Could you check a few things on this model? Use its own coordinates, in mm. A direction names the side the tool comes from. Round coordinates to 2 decimals unless told otherwise and drop trailing zeros. Order: outer loops, then holes, each group sorted by start corner. A loop starts at its lowest first (then second) coordinate and runs counter-clockwise, first axis right, second up. Notation, with made-up numbers: (85, 69.5) - (119, 69.5) arc R20 ccw to (119, 80.5) - close; hole circle Ø7 at (-11.5, 79). An arc over 180 degrees is marked (long way). Return JSON: item names as keys, results as strings. Group by question number.
from build123d import *

# Parameters (mm, degrees)
SKETCH1_W           = 95.25
SKETCH1_H           = 79.375
SKETCH1_W_2         = 73.025
SKETCH1_H_2         = 28.575
BOSS_EXTRUDE1_DEPTH = 3.2
SKETCH2_W           = 95.25
SKETCH2_H           = 79.375
SKETCH2_W_2         = 88.85
SKETCH2_H_2         = 72.975
EXTRUDE_THIN1_DEPTH = 15.24
SKETCH3_R           = 4.064
CUT_EXTRUDE1_DEPTH  = 74.161631893


with BuildPart() as part:
    # Sketch1 → Boss-Extrude1 (new body)
    with BuildSketch(Plane(origin=(0, 0, 0), x_dir=(1, 0, 0), z_dir=(0, 1, 0))):
        with Locations((0, -12.7)):
            Rectangle(SKETCH1_W, SKETCH1_H)
        Rectangle(SKETCH1_W_2, SKETCH1_H_2, mode=Mode.SUBTRACT)
    extrude(amount=BOSS_EXTRUDE1_DEPTH)

    # Sketch2 → Extrude-Thin1 (add)
    with BuildSketch(Plane.XZ):
        with Locations((0, 12.7)):
            Rectangle(SKETCH2_W, SKETCH2_H)
        with Locations((0, 12.7)):
            Rectangle(SKETCH2_W_2, SKETCH2_H_2, mode=Mode.SUBTRACT)
    extrude(amount=EXTRUDE_THIN1_DEPTH)

    # Sketch3 → Cut-Extrude1 (cut, through all)
    with BuildSketch(Plane(origin=(0, 3.2, 0), x_dir=(1, 0, 0), z_dir=(0, 1, 0))):
        with Locations(Location((38.1, -30.1625, 0), (0, 0, 270))):
            Circle(SKETCH3_R)
        with Locations(Location((38.1, -42.8625, 0), (0, 0, 270))):
            Circle(SKETCH3_R)
    extrude(amount=-CUT_EXTRUDE1_DEPTH, mode=Mode.SUBTRACT)


solid = part.part
1) For faces 1 (the flat face through (-36.512, 2, 0)), 2 (the flat face through (-1, 0, 20)), 3 (the flat face through (47.625, -6, 12)), which set-ups out of +Z, -Z, +X, -X, +Y, -Y let a thin tool reach every point of the face, with its end or its side?
2) I want a section at A-A, the plane z = 0.5. List the corners of the cut face in (x, y) for me (1 decimal).
3) We'd pull the mould along Z, two halves only. Please class faces 4 (the flat face through (-1, -6, -26.988)), 5 (the flat face through (-1, 2, -14.288)), 6 (the flat face through (-47.625, -6, 12)): +Z half, -Z half, draft (parallel to the pull), parting line (faces both ways), or undercut.
4) If I drill on line 1 along Z through (x, y) = (31, -1.5); line 2 along X through (y, z) = (-12.75, 4) (3 decimals); line 3 along Y through (x, z) = (37.5, 4.5), over which ranges is the centre line in solid material (lowest first)? Write a range as from..to.
5) I want a section at C-C, the plane x = -24. List the corners of the cut face in (y, z) for me.
6) Will these pins go through, and if not, where does the flat tip stop? pin 1 (8 mm diameter, centred on x = -19.5, z = 34, fed in from -Y); pin 2 (5 mm diameter, centred on x = 38.1, z = 42.86, fed in from +Y).
7) I want a section at B-B, the plane x = 38.1. List the corners of the cut face in (y, z) for me.
8) I want a section at D-D, the plane y = -5. List the corners of the cut face in (x, z) for me (1 decimal), plus the area to 3 significant figures.
Outcome:
{
 "1": {"face 1": "+Y, -Y", "face 2": "-Y", "face 3": "+Z, -Z, +X, +Y, -Y"},
 "2": {"outline": "(-47.6, -15.2) - (-44.4, -15.2) - (-44.4, 0) - (-36.5, 0) - (-36.5, 3.2) - (-47.6, 3.2) - close; (36.5, 0) - (44.4, 0) - (44.4, -15.2) - (47.6, -15.2) - (47.6, 3.2) - (36.5, 3.2) - close"},
 "3": {"face 4": "-Z half", "face 5": "undercut", "face 6": "draft"},
 "4": {"line 1": "-26.99..-23.79, 49.19..52.39", "line 2": "-47.625..-44.425, 44.425..47.625", "line 3": "0..3.2"},
 "5": {"outline": "(-15.24, -26.99) - (3.2, -26.99) - (3.2, -14.29) - (0, -14.29) - (0, -23.79) - (-15.24, -23.79) - close; (-15.24, 49.19) - (0, 49.19) - (0, 14.29) - (3.2, 14.29) - (3.2, 52.39) - (-15.24, 52.39) - close"},
 "6": {"pin 1": "y = 0", "pin 2": "through"},
 "7": {"outline": "(-15.24, -26.99) - (3.2, -26.99) - (3.2, 26.1) - (0, 26.1) - (0, -23.79) - (-15.24, -23.79) - close; (-15.24, 49.19) - (0, 49.19) - (0, 46.93) - (3.2, 46.93) - (3.2, 52.39) - (-15.24, 52.39) - close; (0, 34.23) - (3.2, 34.23) - (3.2, 38.8) - (0, 38.8) - close"},
 "8": {"outline": "(-47.6, -27) - (47.6, -27) - (47.6, 52.4) - (-47.6, 52.4) - close; hole (-44.4, -23.8) - (44.4, -23.8) - (44.4, 49.2) - (-44.4, 49.2) - close", "area": "1,080 mm^2"}
}
